Input: part model. Units: mm. Frame: model coordinates. Face numbers are marked on the shaded views. A direction names the side the tool comes from. Coordinates: 2 decimals unless noted, no trailing zeros. Order: outer loops, then holes, each group sorted by start corner. A loop starts at its lowest first (then second) coordinate and runs counter-clockwise, first axis right, second up. Notation, with made-up numbers: (-22, 42) -> (-3, 42) arc R34 cw to (-3, 78) -> close; hole circle Ø4 at (-6.5, -37.75). An arc over 180 degrees is marked (long way). One line per question, with ' | ' between items.
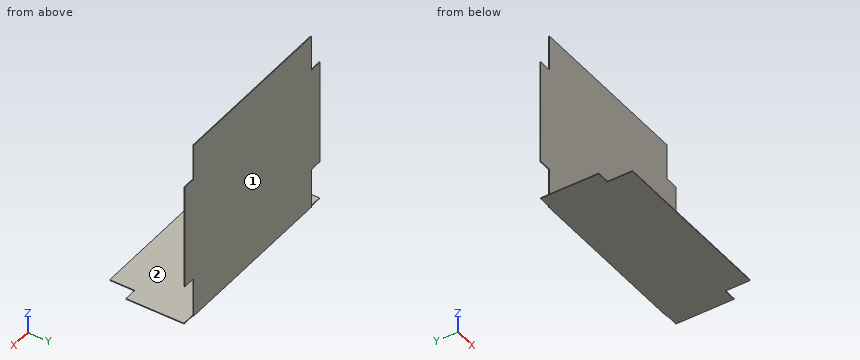
```python
from build123d import *

# Parameters (mm, degrees)
F0_W     = 266.7
F0_H     = 577.85
F1_DEPTH = 317.5
F2_T     = -2.54
F3_W     = 41.275
F3_H     = 114.3
F3_H_2   = 127
F4_DEPTH = 2.54
F5_W     = 41.275
F5_H     = 79.375
F6_DEPTH = 2.541


with BuildPart() as f1:
    # F0 (on Right) → F1 (new body, symmetric)
    with BuildSketch(Plane.YZ):
        Rectangle(F0_W, F0_H)
    extrude(amount=F1_DEPTH, both=True)

    # F2
    f2_openings = [f1.faces().sort_by_distance(p)[0] for p in [
        (0, -133.35, 0),
        (0, 0, 288.925),
        (317.5, 0, 0),
        (-317.5, 0, 0),
    ]]
    offset(amount=F2_T, openings=f2_openings)

    # F3 (on face) → F4 (cut, through all)
    with BuildSketch(Plane(origin=(0, 133.35, 0), x_dir=(-1, 0, 0), z_dir=(0, 1, 0))):
        with Locations((-296.8625, 231.775)):
            Rectangle(F3_W, F3_H)
        with Locations((296.8625, 231.775)):
            Rectangle(F3_W, F3_H)
        with Locations((-296.8625, -225.425)):
            Rectangle(F3_W, F3_H_2)
        with Locations((296.8625, -225.425)):
            Rectangle(F3_W, F3_H_2)
    extrude(amount=-F4_DEPTH, mode=Mode.SUBTRACT)

    # F5 (on face) → F6 (cut, through all)
    with BuildSketch(Plane.XY.offset(-286.385)):
        with Locations((-296.8625, -93.6625)):
            Rectangle(F5_W, F5_H)
        with Locations((296.8625, -93.6625)):
            Rectangle(F5_W, F5_H)
    extrude(amount=-F6_DEPTH, mode=Mode.SUBTRACT)


solid = f1.part
```
1. Cut plane C-C, the plane y = 60. Return loops of the section in (x, z) (3 decimals).
Recorded:
outline: (-317.5, -288.925) -> (317.5, -288.925) -> (317.5, -286.385) -> (-317.5, -286.385) -> close
2. Pin query (flat end, axial travel): pin 1 Ø0.8 at (y, z) = (132.5, 228) entering from +X (3 decimals); pin 2 Ø3 at (x, y) = (306.5, 132) entering from +Z (3 decimals); pin 3 Ø2 at (y, z) = (132, -225) entering from -X (3 decimals). Return the tip coordinate at first contact, or that it passes through.
Recorded:
pin 1: stops at x = 276.225 | pin 2: stops at z = 174.625 | pin 3: stops at x = -276.225
3. Access query for the marked faces 1 and 2. Directions: +Z, -Z, +X, -X, +Y, -Y. A direction counts if a zero-diameter tool reaches every point of the face in a straight line with its end or side. Return the directions, or none.
Recorded:
face 1: +Z, -Z, +X, -X, +Y | face 2: +Z, +X, -X, -Y
4. Cut plane B-B, the plane z = 147. Return loops of the section in (x, y), and give its area (3 significant figures).
Recorded:
outline: (-317.5, 130.81) -> (317.5, 130.81) -> (317.5, 133.35) -> (-317.5, 133.35) -> close | area: 1,610 mm^2
5. Cut plane A-A, the plane x = 188.5. Return loops of the section in (y, z) (3 decimals).
Recorded:
outline: (-133.35, -288.925) -> (133.35, -288.925) -> (133.35, 288.925) -> (130.81, 288.925) -> (130.81, -286.385) -> (-133.35, -286.385) -> close
6. Ray query, line 1 (Z direction, x = 22, y = -110.5) (3 decimals); line 2 (Y direction, x = -56, z = -18.5). Return the intervals inside material, ascending. Write a range as [from, to].
Recorded:
line 1: z = [-288.925, -286.385] | line 2: y = [130.81, 133.35]
